Geometry: final body of the model. Coordinates: model frame, mm. Face numbers are marked on the shaded views. A direction names the side the tool comes from. Give positions to 0.01 mm unless a question says otherwise; leave off trailing zeros. Write each loop counter-clockwise with the first axis right and the second up, starting at its lowest first coordinate (ties: lowest second). Pieces come first, ordered by that corner, then holes. Notation, with made-up numbers: M 70.5,47 L 115.5,47 A19 cw 115.5,73 Z; hole C 46.25,3 d1. An arc over 180 degrees is marked long. Answer as a JSON object with one key per item and string values.
from build123d import *

# Parameters (mm, degrees)
SKETCH_1_W           = 32.5
SKETCH_1_H           = 25.5
EXTRUDE_1_DEPTH      = 3
EXTRUDE_2_DEPTH      = 1.5
SKETCH_5_R           = 1.4
EXTRUDE_3_DEPTH      = 4.5
SKETCH_6_R           = 0.725
EXTRUDE_4_DEPTH      = 1
SKETCH_7_R           = 1
CUT_EXTRUDE_1_DEPTH  = 10
SKETCH_8_R           = 2
CUT_EXTRUDE_2_DEPTH  = 1
FILLET_1_R           = 2
SKETCH_9_R           = 2.65
EXTRUDE_5_DEPTH      = 3.5
SKETCH_11_R          = 1.05
CUT_EXTRUDE_4_DEPTH  = 100
SKETCH_12_R          = 1.41
CUT_EXTRUDE_5_DEPTH  = 5.5
FILLET_2_R           = 0.3
CUT_EXTRUDE_8_DEPTH  = 2
CUT_EXTRUDE_9_DEPTH  = 1.5
EXTRUDE_6_DEPTH      = 6.4
FILLET_3_R           = 2
FILLET_5_R           = 1
FILLET_6_R           = 0.4
CUT_EXTRUDE_13_DEPTH = 1
FILLET_7_R           = 1
SKETCH_22_R          = 1.15
CUT_EXTRUDE_14_DEPTH = 10


with BuildPart() as part:
    # 草图1 → 凸台-拉伸1 (new body)
    with BuildSketch(Plane(origin=(0, 0, 0), x_dir=(1, 0, 0), z_dir=(0, 1, 0))):
        Rectangle(SKETCH_1_W, SKETCH_1_H)
    extrude(amount=EXTRUDE_1_DEPTH)

    # 草图2 → 凸台-拉伸2 (add)
    with BuildSketch(Plane(origin=(0, 3, 0), x_dir=(1, 0, 0), z_dir=(0, 1, 0))):
        Polygon((-5.35, 5.35), (5.35, 5.35), (5.35, -7.55), (4.35, -7.55), (4.35, 4.35), (-4.35, 4.35), (-4.35, -7.55), (-5.35, -7.55), align=None)
    extrude(amount=EXTRUDE_2_DEPTH)

    # 草图5 → 凸台-拉伸3 (add)
    with BuildSketch(Plane(origin=(0, 3, 0), x_dir=(1, 0, 0), z_dir=(0, 1, 0))):
        with Locations(Location((12.5, 5.5, 0), (0, 0, 270))):
            Circle(SKETCH_5_R)
        with Locations(Location((12.5, -5.5, 0), (0, 0, 90))):
            Circle(SKETCH_5_R)
        with Locations(Location((-12.5, -5.5, 0), (0, 0, 270))):
            Circle(SKETCH_5_R)
        with Locations(Location((-12.5, 5.5, 0), (0, 0, 90))):
            Circle(SKETCH_5_R)
    extrude(amount=EXTRUDE_3_DEPTH)

    # 草图6 → 凸台-拉伸4 (add)
    with BuildSketch(Plane(origin=(0, 7.5, 0), x_dir=(1, 0, 0), z_dir=(0, 1, 0))):
        with Locations(Location((-12.5, -5.5, 0), (0, 0, 270))):
            Circle(SKETCH_6_R)
        with Locations(Location((-12.5, 5.5, 0), (0, 0, 270))):
            Circle(SKETCH_6_R)
        with Locations(Location((12.5, 5.5, 0), (0, 0, 270))):
            Circle(SKETCH_6_R)
        with Locations(Location((12.5, -5.5, 0), (0, 0, 270))):
            Circle(SKETCH_6_R)
    extrude(amount=EXTRUDE_4_DEPTH)

    # 草图7 → 切除-拉伸1 (cut)
    with BuildSketch(Plane(origin=(0, 3, 0), x_dir=(1, 0, 0), z_dir=(0, 1, 0))):
        with Locations(Location((13.5, 10, 0), (0, 0, 270))):
            Circle(SKETCH_7_R)
        with Locations(Location((-13.5, 10, 0), (0, 0, 270))):
            Circle(SKETCH_7_R)
        with Locations(Location((-13.5, -10, 0), (0, 0, 270))):
            Circle(SKETCH_7_R)
        with Locations(Location((13.5, -10, 0), (0, 0, 270))):
            Circle(SKETCH_7_R)
    extrude(amount=-CUT_EXTRUDE_1_DEPTH, mode=Mode.SUBTRACT)

    # 草图8 → 切除-拉伸2 (cut)
    with BuildSketch(Plane.XZ):
        with Locations(Location((-13.5, 10, 0), (0, 0, 270))):
            Circle(SKETCH_8_R)
        with Locations(Location((13.5, 10, 0), (0, 0, 270))):
            Circle(SKETCH_8_R)
        with Locations(Location((13.5, -10, 0), (0, 0, 270))):
            Circle(SKETCH_8_R)
        with Locations(Location((-13.5, -10, 0), (0, 0, 270))):
            Circle(SKETCH_8_R)
    extrude(amount=-CUT_EXTRUDE_2_DEPTH, mode=Mode.SUBTRACT)

    # 圆角1
    fillet_1_edges = [part.edges().sort_by_distance(p)[0] for p in [
        (16.25, 1.5, 12.75),
        (-16.25, 1.5, 12.75),
        (-16.25, 1.5, -12.75),
        (16.25, 1.5, -12.75),
    ]]
    fillet(fillet_1_edges, radius=FILLET_1_R)

    # 草图9 → 凸台-拉伸5 (add)
    with BuildSketch(Plane(origin=(0, 3, 0), x_dir=(1, 0, 0), z_dir=(0, 1, 0))):
        with Locations(Location((8.5, 7.75, 0), (0, 0, 270))):
            Circle(SKETCH_9_R)
        with Locations(Location((-8.5, 7.75, 0), (0, 0, 90))):
            Circle(SKETCH_9_R)
        with Locations(Location((-8.5, -7.75, 0), (0, 0, 270))):
            Circle(SKETCH_9_R)
        with Locations(Location((8.5, -7.75, 0), (0, 0, 90))):
            Circle(SKETCH_9_R)
    extrude(amount=EXTRUDE_5_DEPTH)

    # 草图11 → 切除-拉伸4 (cut)
    with BuildSketch(Plane(origin=(0, 6.5, 0), x_dir=(1, 0, 0), z_dir=(0, 1, 0))):
        with Locations(Location((-8.5, 7.75, 0), (0, 0, 270))):
            Circle(SKETCH_11_R)
        with Locations(Location((-8.5, -7.75, 0), (0, 0, 270))):
            Circle(SKETCH_11_R)
        with Locations(Location((8.5, -7.75, 0), (0, 0, 270))):
            Circle(SKETCH_11_R)
        with Locations(Location((8.5, 7.75, 0), (0, 0, 270))):
            Circle(SKETCH_11_R)
    extrude(amount=-CUT_EXTRUDE_4_DEPTH, mode=Mode.SUBTRACT)

    # 草图12 → 切除-拉伸5 (cut)
    with BuildSketch(Plane(origin=(0, 6.5, 0), x_dir=(1, 0, 0), z_dir=(0, 1, 0))):
        with Locations(Location((-8.5, 7.75, 0), (0, 0, 270))):
            Circle(SKETCH_12_R)
        with Locations(Location((8.5, 7.75, 0), (0, 0, 270))):
            Circle(SKETCH_12_R)
        with Locations(Location((-8.5, -7.75, 0), (0, 0, 270))):
            Circle(SKETCH_12_R)
        with Locations(Location((8.5, -7.75, 0), (0, 0, 270))):
            Circle(SKETCH_12_R)
    extrude(amount=-CUT_EXTRUDE_5_DEPTH, mode=Mode.SUBTRACT)

    # 圆角2
    fillet_2_edges = [part.edges().sort_by_distance(p)[0] for p in [
        (-12.5, 8.5, 4.775),
        (-12.5, 8.5, -6.225),
        (12.5, 8.5, -6.225),
        (12.5, 8.5, 4.775),
    ]]
    fillet(fillet_2_edges, radius=FILLET_2_R)

    # 草图15 → 切除-拉伸8 (cut)
    with BuildSketch(Plane(origin=(0, 3, 0), x_dir=(1, 0, 0), z_dir=(0, 1, 0))):
        Polygon((-4.35, 4.35), (4.35, 4.35), (4.35, -7.55), (3.2, -7.55), (3.2, -12.75), (-3.2, -12.75), (-3.2, -7.55), (-4.35, -7.55), align=None)
    extrude(amount=-CUT_EXTRUDE_8_DEPTH, mode=Mode.SUBTRACT)

    # 草图17 → 切除-拉伸9 (cut)
    with BuildSketch(Plane(origin=(0, 4.5, 0), x_dir=(1, 0, 0), z_dir=(0, 1, 0))):
        Polygon((-4.35, -7.55), (-4.35, 4.35), (4.35, 4.35), (4.35, -7.55), (5.35, -7.55), (5.35, 5.35), (-5.35, 5.35), (-5.35, -7.55), align=None)
    extrude(amount=-CUT_EXTRUDE_9_DEPTH, mode=Mode.SUBTRACT)

    # 草图18 → 凸台-拉伸6 (add)
    with BuildSketch(Plane.ZY.offset(-3.2)):
        Polygon((12.75, 1), (9.75, 1), (12.25, 2.6), (12.75, 2.6), align=None)
    extrude(amount=EXTRUDE_6_DEPTH)

    # 圆角3
    fillet_3_edges = [part.edges().sort_by_distance(p)[0] for p in [
        (0, 1, 9.75),
    ]]
    fillet(fillet_3_edges, radius=FILLET_3_R)

    # 圆角5
    fillet_5_edges = [part.edges().sort_by_distance(p)[0] for p in [
        (0, 2.6, 12.25),
    ]]
    fillet(fillet_5_edges, radius=FILLET_5_R)

    # 圆角6
    fillet_6_edges = [part.edges().sort_by_distance(p)[0] for p in [
        (3.2, 2, 7.55),
        (-3.2, 2, 7.55),
    ]]
    fillet(fillet_6_edges, radius=FILLET_6_R)

    # 草图21 → 切除-拉伸13 (cut)
    with BuildSketch(Plane.XZ):
        Polygon((-13.5, -7.3), (-10.8, -7.3), (-10.8, -12.75), (-16.25, -12.75), (-16.25, -7.3), align=None)
        Polygon((16.25, -12.75), (16.25, -7.3), (13.5, -7.3), (10.8, -7.3), (10.8, -12.75), align=None)
        Polygon((16.25, 12.75), (16.25, 7.3), (13.5, 7.3), (10.8, 7.3), (10.8, 12.75), align=None)
        Polygon((-10.8, 12.75), (-16.25, 12.75), (-16.25, 7.3), (-13.5, 7.3), (-10.8, 7.3), align=None)
    extrude(amount=-CUT_EXTRUDE_13_DEPTH, mode=Mode.SUBTRACT)

    # 圆角7
    fillet_7_edges = [part.edges().sort_by_distance(p)[0] for p in [
        (-16.25, 0.5, 7.3),
        (-10.8, 0.5, 12.75),
        (-10.8, 0.5, 7.3),
        (10.8, 0.5, 12.75),
        (16.25, 0.5, 7.3),
        (10.8, 0.5, 7.3),
        (16.25, 0.5, -7.3),
        (10.8, 0.5, -12.75),
        (10.8, 0.5, -7.3),
        (-10.8, 0.5, -12.75),
        (-16.25, 0.5, -7.3),
        (-10.8, 0.5, -7.3),
    ]]
    fillet(fillet_7_edges, radius=FILLET_7_R)

    # 草图22 → 切除-拉伸14 (cut)
    with BuildSketch(Plane.XZ.offset(-1)):
        with Locations(Location((13.5, -10, 0), (0, 0, 270))):
            Circle(SKETCH_22_R)
        with Locations(Location((13.5, 10, 0), (0, 0, 270))):
            Circle(SKETCH_22_R)
        with Locations(Location((-13.5, 10, 0), (0, 0, 270))):
            Circle(SKETCH_22_R)
        with Locations(Location((-13.5, -10, 0), (0, 0, 270))):
            Circle(SKETCH_22_R)
    extrude(amount=-CUT_EXTRUDE_14_DEPTH, mode=Mode.SUBTRACT)


solid = part.part
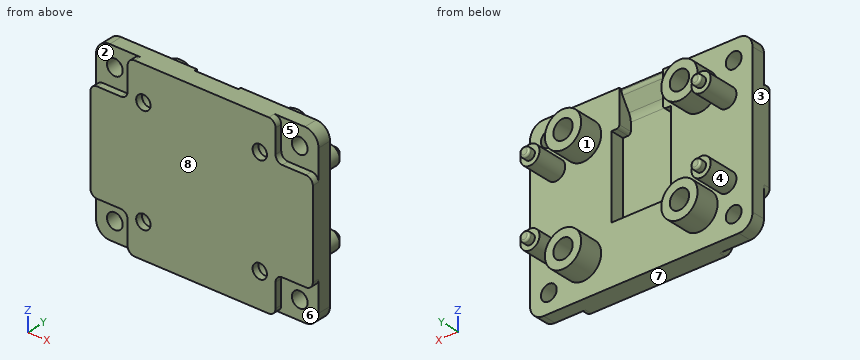
1) Cut plane D-D on x = -6.5. Return loops of the section in (y, z), and give its area (3 significant figures).
Geometry check:
{"outline": "M 0,-12.75 L 3,-12.75 L 3,-9.49 L 6.5,-9.49 L 6.5,-6.01 L 3,-6.01 L 3,6.01 L 6.5,6.01 L 6.5,9.49 L 3,9.49 L 3,12.75 L 0,12.75 Z", "area": "101 mm2"}
2) Cut plane C-C on x = 2. Return loops of the section in (y, z), and give its area (3 significant figures).
Geometry check:
{"outline": "M 0,-12.75 L 3,-12.75 L 3,-4.35 L 1,-4.35 L 1,9.16 A2 cw 1.32,10.24 L 2.44,12 A1 ccw 2.6,12.54 L 2.6,12.75 L 0,12.75 Z", "area": "45.1 mm2"}
3) Contact query for flat-ended pins moving along their axis: P1, Ø0.8, axis at y = 0.5, z = -9.5, coming from the +X side; P2, Ø2, axis at y = 5.5, z = -3, coming from the +X side; P3, Ø3.5, axis at x = -8.5, z = 7.75, coming from the -Y side; P4, Ø2.5, axis at x = 9, z = 8, coming from the +Y side. Output: stop coordinate, or through.
Geometry check:
{"P1": "stops at x = 10.8", "P2": "passes through", "P3": "stops at y = 0", "P4": "stops at y = 6.5"}
4) Cut plane B-B on x = 8.5. Return loops of the section in (y, z), and give its area (3 significant figures).
Geometry check:
{"outline": "M 0,-12.75 L 3,-12.75 L 3,-10.4 L 6.5,-10.4 L 6.5,-9.16 L 1,-9.16 L 1,-8.8 L 0,-8.8 Z; M 0,-6.7 L 1,-6.7 L 1,-6.34 L 6.5,-6.34 L 6.5,-5.1 L 3,-5.1 L 3,5.1 L 6.5,5.1 L 6.5,6.34 L 1,6.34 L 1,6.7 L 0,6.7 Z; M 0,8.8 L 1,8.8 L 1,9.16 L 6.5,9.16 L 6.5,10.4 L 3,10.4 L 3,12.75 L 0,12.75 Z", "area": "78.4 mm2"}
5) Cut plane A-A on y = 3.75. Give the number of separate pieces and of enclosed holes in the cut face, and give its area (3 significant figures).
Geometry check:
{"separate pieces": "8", "enclosed holes": "4", "area": "87.9 mm2"}
6) Set-up query: the marked faces 4, 5, 6, 7 and 8. Return all of +Z, -Z, +X, -X, +Y, -Y with unobstructed straight access to the full face (end or side cutting, diameter ignored); none if empty.
Geometry check:
{"face 4": "+Y", "face 5": "+Z, +X, -Y", "face 6": "-Z, +X, -Y", "face 7": "-Z, +X, -X, +Y, -Y", "face 8": "+Z, -Z, +X, -X, -Y"}
7) Line query: line 1 (X direction, y = 3.85, z = -7.75); line 2 (X direction, y = 1.8, z = -10); line 3 (Z direction, x = -9.5, y = 4.5). Output: solid intervals per line, ascending. Write a range as from..to.
Geometry check:
{"line 1": "x = -11.15..-9.91, -7.09..-5.85, 5.85..7.09, 9.91..11.15", "line 2": "x = -16.25..-14.65, -12.35..12.35, 14.65..16.25", "line 3": "z = -10.2..-8.74, -6.76..-5.3, 5.3..6.76, 8.74..10.2"}
8) Pull-direction query (X, two-part tool) for the marked faces 1, 2 and 3; classes: pulls with the +X half, pulls with the -X half, needs draft (parallel to the pull), parting line crosses it, or undercut.
Geometry check:
{"face 1": "undercut", "face 2": "needs draft", "face 3": "pulls with the -X half"}
